Geometry check sheet. Reference: the model listing, model coordinates, mm. Face numbers are marked on the shaded views. A direction names the side the tool comes from. Round coordinates to 2 decimals unless told otherwise and drop trailing zeros. Write each loop counter-clockwise with the first axis right and the second up, starting at its lowest first coordinate (ties: lowest second). Pieces come first, ordered by that corner, then holes. Notation, with made-up numbers: (19, 83.25) -> (52, 83.25) arc R22 cw to (52, 121.25) -> close; hole circle Ø5 at (11.25, -38.5). An arc over 180 degrees is marked (long way). Put each result on its own line as item: value. Start each with the question number.
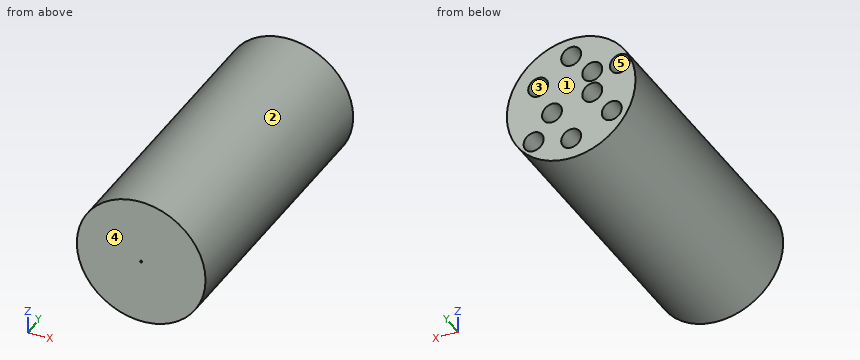
from build123d import *

# Parameters (mm, degrees)
F0_R     = 16.3722286136
F1_DEPTH = 73.152
F3_D     = 0.508
F3_DEPTH = 12.7
F3_TIP   = 0.1526185972
F5_D     = 5.08
F5_DEPTH = 38.1
F5_TIP   = 1.5261859723


with BuildPart() as f1:
    # F0 (on Front) → F1 (new body)
    with BuildSketch(Plane.XZ):
        Circle(F0_R)
    extrude(amount=F1_DEPTH)

    # F3
    with Locations(Plane.XZ.offset(73.152)):
        with Locations((0, 0)):
            Hole(F3_D / 2, depth=F3_DEPTH)
            with Locations((0, 0, -(F3_DEPTH + F3_TIP / 2))):  # 118° drill point
                Cone(0, F3_D / 2, F3_TIP, mode=Mode.SUBTRACT)

    # F5
    with Locations(Plane(origin=(0, 0, 0), x_dir=(1, 0, 0), z_dir=(0, 1, 0))):
        with Locations((-12.3842703179, -5.7045519352), (-5.3632836789, -5.7045519352), (0, -11.5553746), (8.3861500025, -5.7045519352), (-5.3632836789, 0), (4.8756562173, 2.4865996093), (9.556314908, 8.9225051925), (0, 10.9702926129), (-10.3364828974, 6.5821758471)):
            Hole(F5_D / 2, depth=F5_DEPTH)
            with Locations((0, 0, -(F5_DEPTH + F5_TIP / 2))):  # 118° drill point
                Cone(0, F5_D / 2, F5_TIP, mode=Mode.SUBTRACT)


solid = f1.part
(1) Sectioned sample at C-C (y = -43.5). Record the cut outline in (x, z).
(2) Go/stop test with flat-tipped pins: pin 1 Ø10 at (y, z) = (-33.5, 8) entering from -X (3 decimals); pin 2 Ø4 at (x, z) = (0, -10.97) entering from +Y; pin 3 Ø4 at (y, z) = (-34.5, -9.5) entering from -X. Record where each tip stops, or that it passes through.
(3) Sectioned sample at A-A (y = -65). Record the cut outline in (x, z), and give its area (3 significant figures).
(4) Set-up check for the marked faces 4 and 5: record each of +Z, -Z, +X, -X, +Y, -Y from which the full face is reachable in a straight line by a thin tool's end or side.
(5) Mould release check, pull along X, two halves, no side actions. Record for the marked faces 1, 2 and 3: +X half, -X half, draft (parallel to the pull), parting line (faces both ways), or undercut.
(6) Material ranges on L1, parallel to Z at x = -0.5, y = -36.5; L2, parallel to X at y = -32.5, z = -0.5; L3, parallel to Z at x = -7.5, y = -15, recorded low to high. Write a range as from..to.
(7) Sectioned sample at B-B (y = -7). State how many separate pieces and enclosed holes the cut face has, and give its area (3 significant figures).
Found:
1. outline: circle Ø32.74 at (0, 0)
2. pin 1: x = -16.095
2. pin 2: y = -38.42
2. pin 3: x = -14.55
3. outline: circle Ø32.74 at (0, 0); hole circle Ø0.51 at (0, 0)
3. area: 842 mm2
4. face 4: +Z, -Z, +X, -X, -Y
4. face 5: +Y
5. face 1: draft
5. face 2: parting line
5. face 3: undercut
6. L1: -16.36..-13.46, -8.48..9.07, 14.05..16.36
6. L2: -16.36..-7.85, -2.87..3.29, 6.46..16.36
6. L3: -14.55..-1.37, 1.37..4.33, 7.08..14.55
7. separate pieces: 1
7. enclosed holes: 9
7. area: 660 mm2
